Geometry check sheet. Reference: the model listing, model coordinates, mm. A direction names the side the tool comes from. Give positions to 0.01 mm unless a question says otherwise; leave off trailing zeros. Order: outer loops, then holes, each group sorted by start corner. A loop starts at its lowest first (then second) coordinate and runs counter-clockwise, first axis right, second up. Notation, with made-up numbers: M -0.75,-30 L 30.25,-30 A11 ccw 30.25,-20 Z; hole C 68.25,30 d6. An arc over 180 degrees is marked long. One line per question, with ' | ' between items. Start each with the question number.
from build123d import *

# Parameters (mm, degrees)
SKETCH1_W               = 42.3
SKETCH1_H               = 42.3
BOSS_EXTRUDE1_DEPTH     = 9.6
CHAMFER1_SIZE           = 4
BOSS_EXTRUDE2_DEPTH     = 18.8
BOSS_EXTRUDE3_DEPTH     = 9.6
SKETCH4_R               = 11
SKETCH4_R_2             = 5
BOSS_EXTRUDE4_DEPTH     = 2
SKETCH5_R               = 2.5
BOSS_EXTRUDE5_DEPTH     = 20
SKETCH8_R               = 1.5
CUT_EXTRUDE1_DEPTH      = 4
MIRROR2_COPY_1_SKETCH_R = 1.5
MIRROR2_COPY_1_DEPTH    = 4
MIRROR3_COPY_1_SKETCH_R = 1.5
MIRROR3_COPY_1_DEPTH    = 4
MIRROR3_COPY_2_SKETCH_R = 1.5
MIRROR3_COPY_2_DEPTH    = 4
MIRROR3_COPY_3_SKETCH_R = 1.5
MIRROR3_COPY_3_DEPTH    = 4
SKETCH9_W               = 16
SKETCH9_H               = 9.6
BOSS_EXTRUDE6_DEPTH     = 4
SKETCH10_W              = 16
SKETCH10_H              = 6.4
BOSS_EXTRUDE7_DEPTH     = 2
SKETCH11_W              = 15
SKETCH11_H              = 5.4
CUT_EXTRUDE2_DEPTH      = 4


with BuildPart() as part:
    # Sketch1 → Boss-Extrude1 (new body)
    with BuildSketch(Plane(origin=(0, 0, 0), x_dir=(1, 0, 0), z_dir=(0, 1, 0))):
        Rectangle(SKETCH1_W, SKETCH1_H)
    extrude(amount=BOSS_EXTRUDE1_DEPTH)

    # Chamfer1
    chamfer1_edges = [part.edges().sort_by_distance(p)[0] for p in [
        (-21.15, 4.8, -21.15),
        (21.15, 4.8, -21.15),
        (21.15, 4.8, 21.15),
        (-21.15, 4.8, 21.15),
    ]]
    chamfer(chamfer1_edges, length=CHAMFER1_SIZE)

    # Sketch2 → Boss-Extrude2 (add)
    with BuildSketch(Plane(origin=(0, 9.6, 0), x_dir=(1, 0, 0), z_dir=(0, 1, 0))):
        Polygon((13.75, -21.15), (21.15, -13.74318557), (21.15, 13.74318557), (13.75, 21.15), (-13.75, 21.15), (-21.15, 13.74318557), (-21.15, -13.74318557), (-13.75, -21.15), align=None)
    extrude(amount=BOSS_EXTRUDE2_DEPTH)

    # Sketch3 → Boss-Extrude3 (add)
    with BuildSketch(Plane(origin=(0, 28.4, 0), x_dir=(1, 0, 0), z_dir=(0, 1, 0))):
        Polygon((17.15, 21.15), (-17.15, 21.15), (-21.15, 17.15), (-21.15, -17.15), (-17.15, -21.15), (17.15, -21.15), (21.15, -17.15), (21.15, 17.15), align=None)
    extrude(amount=BOSS_EXTRUDE3_DEPTH)

    # Sketch4 → Boss-Extrude4 (add)
    with BuildSketch(Plane(origin=(0, 38, 0), x_dir=(1, 0, 0), z_dir=(0, 1, 0))):
        with Locations(Location((0, 0, 0), (0, 0, 270))):
            Circle(SKETCH4_R)
        with Locations(Location((0, 0, 0), (0, 0, 270))):
            Circle(SKETCH4_R_2, mode=Mode.SUBTRACT)
    extrude(amount=BOSS_EXTRUDE4_DEPTH)

    # Sketch5 → Boss-Extrude5 (add)
    with BuildSketch(Plane(origin=(0, 38, 0), x_dir=(1, 0, 0), z_dir=(0, 1, 0))):
        with Locations(Location((0, 0, 0), (0, 0, 270))):
            Circle(SKETCH5_R)
    extrude(amount=BOSS_EXTRUDE5_DEPTH)

    # Sketch8 → Cut-Extrude1 (cut)
    with BuildSketch(Plane(origin=(0, 38, 0), x_dir=(1, 0, 0), z_dir=(0, 1, 0))):
        with Locations(Location((15.5, -15.5, 0), (0, 0, 270))):
            Circle(SKETCH8_R)
    cut_extrude1 = extrude(amount=-CUT_EXTRUDE1_DEPTH, mode=Mode.SUBTRACT)

    # Mirror1: Cut-Extrude1 across plane
    add(cut_extrude1.mirror(Plane.XY), mode=Mode.SUBTRACT)

    # Mirror2: Cut-Extrude1 across plane
    add(cut_extrude1.mirror(Plane(origin=(0, 0, 0), x_dir=(0, 0, 1), z_dir=(1, 0, 0))), mode=Mode.SUBTRACT)

    # Mirror2 copy 1 sketch → Mirror2 copy 1 (cut)
    with BuildSketch(Plane(origin=(0, 38, 0), x_dir=(-1, 0, 0), z_dir=(0, 1, 0))):
        with Locations(Location((15.5, -15.5, 0), (0, 0, 270))):
            Circle(MIRROR2_COPY_1_SKETCH_R)
    extrude(amount=-MIRROR2_COPY_1_DEPTH, mode=Mode.SUBTRACT)

    # Mirror3: Cut-Extrude1 across plane
    add(cut_extrude1.mirror(Plane.ZX.offset(19)), mode=Mode.SUBTRACT)

    # Mirror3 copy 1 sketch → Mirror3 copy 1 (cut)
    with BuildSketch(Plane.XZ):
        with Locations(Location((15.5, -15.5, 0), (0, 0, 270))):
            Circle(MIRROR3_COPY_1_SKETCH_R)
    extrude(amount=-MIRROR3_COPY_1_DEPTH, mode=Mode.SUBTRACT)

    # Mirror3 copy 2 sketch → Mirror3 copy 2 (cut)
    with BuildSketch(Plane(origin=(0, 0, 0), x_dir=(-1, 0, 0), z_dir=(0, -1, 0))):
        with Locations(Location((15.5, -15.5, 0), (0, 0, 270))):
            Circle(MIRROR3_COPY_2_SKETCH_R)
    extrude(amount=-MIRROR3_COPY_2_DEPTH, mode=Mode.SUBTRACT)

    # Mirror3 copy 3 sketch → Mirror3 copy 3 (cut)
    with BuildSketch(Plane(origin=(0, 0, 0), x_dir=(-1, 0, 0), z_dir=(0, -1, 0))):
        with Locations((15.5, 15.5)):
            Circle(MIRROR3_COPY_3_SKETCH_R)
    extrude(amount=-MIRROR3_COPY_3_DEPTH, mode=Mode.SUBTRACT)

    # Sketch9 → Boss-Extrude6 (add)
    with BuildSketch(Plane(origin=(0, 0, -21.15), x_dir=(-1, 0, 0), z_dir=(0, 0, -1))):
        with Locations((0, 4.8)):
            Rectangle(SKETCH9_W, SKETCH9_H)
    extrude(amount=BOSS_EXTRUDE6_DEPTH)

    # Sketch10 → Boss-Extrude7 (add)
    with BuildSketch(Plane(origin=(0, 0, -25.15), x_dir=(-1, 0, 0), z_dir=(0, 0, -1))):
        with Locations((0, 6.4)):
            Rectangle(SKETCH10_W, SKETCH10_H)
    extrude(amount=BOSS_EXTRUDE7_DEPTH)

    # Sketch11 → Cut-Extrude2 (cut)
    with BuildSketch(Plane(origin=(0, 0, -27.15), x_dir=(-1, 0, 0), z_dir=(0, 0, -1))):
        with Locations((0, 6.4)):
            Rectangle(SKETCH11_W, SKETCH11_H)
    extrude(amount=-CUT_EXTRUDE2_DEPTH, mode=Mode.SUBTRACT)


solid = part.part
Item 1: Mould release check, pull along Y, two halves, no side actions. Record for faces 4 (the cylindrical face through (-4.88, 38.99, -1.08)), 5 (the flat face through (0, 0, -2)), 6 (the flat face through (18, 9.6, -18)): released by +Y, released by -Y, zero draft, split by the parting line, or undercut.
Item 2: Depth check by flat-ended pin: pin 1 (2 mm diameter, centred on x = 18, z = -18, fed in from +Y); pin 2 (1 mm diameter, centred on x = 12, y = 12.5, fed in from -Z); pin 3 (2.5 mm diameter, centred on x = -15.5, z = -15.5, fed in from -Y). Enter the tip coordinate at first touch or a pass-through.
Item 3: Material ranges on line 1 along X through (y, z) = (36.2, 15.5); line 2 along X through (y, z) = (39, 0), recorded low to high.
Item 4: Cross-section at D-D, the plane y = 27. Record the cut outline in (x, z).
Item 5: Cross-section at A-A, the plane y = 36. Record the cut outline in (x, z), plus the area to 3 significant figures.
Item 6: Cross-section at C-C, the plane x = 0. Record the cut outline in (y, z).
Item 7: Cross-section at B-B, the plane z = -24. Record the cut outline in (x, y), plus the area to 3 significant figures.
Item 8: Set-up check for faces 1 (the flat face through (0, 9.1, -25)), 2 (the flat face through (-18, 28.4, 18)), 3 (the flat face through (16, 4, -15)): record each of +Z, -Z, +X, -X, +Y, -Y from which the full face is reachable in a straight line by a thin tool's end or side.
Outcome:
1) face 4: zero draft | face 5: released by -Y | face 6: undercut
2) pin 1: stops at y = 38 | pin 2: stops at z = -21.15 | pin 3: stops at y = 4
3) line 1: x = -21.15 to -17, -14 to 14, 17 to 21.15 | line 2: x = -11 to -5, -2.5 to 2.5, 5 to 11
4) outline: M -21.15,-13.74 L -13.75,-21.15 L 13.75,-21.15 L 21.15,-13.74 L 21.15,13.74 L 13.75,21.15 L -13.75,21.15 L -21.15,13.74 Z
5) outline: M -21.15,-17.15 L -17.15,-21.15 L 17.15,-21.15 L 21.15,-17.15 L 21.15,17.15 L 17.15,21.15 L -17.15,21.15 L -21.15,17.15 Z; hole C -15.5,-15.5 d3; hole C -15.5,15.5 d3; hole C 15.5,-15.5 d3; hole C 15.5,15.5 d3 | area: 1,730 mm²
6) outline: M 0,-25.15 L 3.2,-25.15 L 3.2,-27.15 L 3.7,-27.15 L 3.7,-23.15 L 9.1,-23.15 L 9.1,-27.15 L 9.6,-27.15 L 9.6,-21.15 L 38,-21.15 L 38,-11 L 40,-11 L 40,-5 L 38,-5 L 38,-2.5 L 58,-2.5 L 58,2.5 L 38,2.5 L 38,5 L 40,5 L 40,11 L 38,11 L 38,21.15 L 0,21.15 Z
7) outline: M -8,0 L 8,0 L 8,9.6 L -8,9.6 Z; hole M -7.5,3.7 L 7.5,3.7 L 7.5,9.1 L -7.5,9.1 Z | area: 72.6 mm²
8) face 1: -Z | face 2: +Z, -X | face 3: -Y
